Autodesk Inventor part; units mm, degrees
ref_plane "Plano de trabalho4" through (-4.5, 0, 0) normal (-1, 0, 0) x (0, 0, 1)
ref_plane "YZ Plane" through (0, 0, 0) normal (1, 0, 0) x (0, 1, 0)
ref_plane "XZ Plane" through (0, 0, 0) normal (0, 1, 0) x (-1, 0, 0)
sketch "Esboço1" plane through (0, 0, 0) normal (0, 0, 1) x (1, 0, 0)
  line L0 (0, 0) -> (0, 30)
  line L1 (0, 3) -> (-8, 3)
  line L2 (0, 0) -> (2.8421, 0)
  circle A0 centre (-4.5, 30) radius 3
  line L3 (-1.5, 30) -> (0, 30)
  line L4 (-7.5, 30) -> (-9, 30)
  line L5 (-8, 3) -> (-8, 6)
  line L6 (-9, 30) -> (-9, 25)
  line L7 (-9, 25) -> (-8, 25)
  arc A1 (-8, 6) -> (-8, 25) centre (-11.8508, 15.5) ccw
  point P0 (0, 15)
  point P1 (-1.6, 15.5)
  dimension "d1" = 3
  dimension "d3" = 6
  dimension "d4" = 1.5
  dimension "d7" = 1.5
  dimension "d15" = 8
  dimension "d79" = 0
  dimension "d80" = 0
  dimension "d81" = 30
  dimension "d93" = 5
  dimension "d94" = 3
  dimension "d95" = 1.6
revolve "Revolução1" add sketch "Esboço1" angle 360 about axis through (0, 0, 0) along (1, 0, 0) contours L1 L5 A1 L7 L6 L4 A0 L3 L0
sketch "Esboço3" plane through (-8, 0, 0) normal (-1, 0, 0) x (0, -1, 0)
  circle A0 centre (0, 0) radius 3
  arc A1 (-2.2361, -2) -> (0, -3) centre (0, 0) ccw
  arc A2 (-2.2361, -2) -> (2.2361, -2) centre (0, 0) ccw
  line L0 (-2.2361, 2) -> (2.2361, 2)
  line L1 (-2.2361, -2) -> (2.2361, -2)
  dimension "d84" = 4
sketch "Esboço6" plane through (-8, 0, 0) normal (-1, 0, 0) x (0, -1, 0)
  circle A0 centre (0, 0) radius 6
  circle A1 centre (0, 0) radius 3
ref_plane "Plano de trabalho4" through (-4.5, 0, 0) normal (-1, 0, 0) x (0, 0, 1)
extrude "Extrusão9" add sketch "Esboço3" along normal blind 2 and the other way blind 8 contours L0 A0 | A0 L1
extrude "Extrusão10" add sketch "Esboço6" along normal blind 2
fillet "Arredondamento13" radius 2 1 edges at (-10, 6, 0)
equation "\"d23\" = d22"
properties part number "Rodinha-01"
The listing builds one solid part. Answer for the finished solid, in the listing's coordinates (mm). A direction names the side the tool comes from. Round coordinates to 2 decimals unless told otherwise and drop trailing zeros. Write each loop counter-clockwise with the first axis right and the second up, starting at its lowest first coordinate (ties: lowest second). Pieces come first, ordered by that corner, then holes. Notation, with made-up numbers: (67, 37.25) - (120, 37.25) arc R29 cw to (120, 69.25) - close; hole circle Ø6 at (-31, 20.5). An arc over 180 degrees is marked (long way). Use a Markdown table: item, result. Add a question column.
1. The part is cut by section B-B (x = -3.5). Write down the section's boundary in (y, z).
2. Consider line 1 (Z direction, x = -8.25, y = 0); line 2 (Z direction, x = -8.65, y = 0); line 3 (X direction, y = -7.5, z = -25). Determine where each line is inside the solid, lowest interval first.
3. Flat-ended cylindrical pins translate along their axes: P1, Ø2, axis at x = -3.5, z = -15, coming from the +Y side; P2, Ø1.3, axis at x = -7, y = 0, coming from the -Z side; P3, Ø6, axis at x = -7, y = 14.5, coming from the -Z side. Find the tip coordinate at first contact, or state that the pin passes through.
4. A tool of negligible diameter and unlimited length cuts with its end or side. For faces 4 (the face through (-10, 0, -3)), 5 (the face through (-5, 3, 0)), 6 (the face through (-8.493, 23.846, 7.509)), from which of +Z, -Z, +X, -X, +Y, -Y can it reach the whole face along a straight path? Write none if from no direction.
5. For a pull along Z with two mould halves and no side action, classify faces 1 (the face through (-9, -7, 25)), 2 (the face through (-8.26, -29.97, -1.32)), 3 (the face through (-5, -3, 0)) as +Z half, -Z half, draft (parallel to the pull), parting line (faces both ways), or undercut.
Reported:
| question | item | result |
|---|---|---|
| 1 | outline | circle Ø54.34 at (0, 0); circle Ø19.11 at (0, 0); hole circle Ø42.89 at (0, 0); hole (-2.24, -2) - (2.24, -2) arc R3 ccw to (2.24, 2) - (-2.24, 2) arc R3 ccw to start |
| 2 | line 1 | -30 to -25, -5.98 to -2, 2 to 5.98, 25 to 30 |
| 2 | line 2 | -30 to -25, -5.89 to -2, 2 to 5.89, 25 to 30 |
| 2 | line 3 | -9 to 0 |
| 3 | P1 | y = 23.55 |
| 3 | P2 | z = -30 |
| 3 | P3 | z = -27.69 |
| 4 | face 4 | +Z, -Z, -X, +Y, -Y |
| 4 | face 5 | +X, -X |
| 4 | face 6 | -X |
| 5 | face 1 | draft |
| 5 | face 2 | parting line |
| 5 | face 3 | undercut |
